Geometry check sheet. Reference: the model listing, model coordinates, mm. A direction names the side the tool comes from. Coordinates: 2 decimals unless noted, no trailing zeros. Order: outer loops, then holes, each group sorted by start corner. A loop starts at its lowest first (then second) coordinate and runs counter-clockwise, first axis right, second up. Notation, with made-up numbers: M -29.75,35 L -16.75,35 A22 ccw -16.75,56 Z; hole C 66,63.5 d11. An arc over 180 degrees is marked long. One line per item, written item: value. Start each with the question number.
1) Sectioned sample at D-D, the plane y = -1.5. Enter the section's corners in (x, z), then the cut area to 3 significant figures.
2) Draft check along Y on faces 1 (the flat face through (19, -22, 9.525)), 2 (the flat face through (32.6, -17.1, 11)), 3 (the flat face through (23.55, -3.13, 19.32)). Enter one of: pulls with the +Y half, pulls with the -Y half, needs draft (parallel to the pull), parting line crosses it, or undercut.
3) Sectioned sample at B-B, the plane x = 20.5. State how many separate pieces and enclosed holes the cut face has, then the cut area to 3 significant figures.
4) Thickness scan on L1, parallel to Y at x = 13, z = 27; L2, parallel to Y at x = 5, z = 23.5; L3, parallel to X at y = -16.5, z = 21. Record the ranges inside material, lowest first. Write a range as from..to.
5) Sectioned sample at C-C, the plane z = 35. Enter the section's corners in (x, y), then the cut area to 3 significant figures.
6) Sectioned sample at A-A, the plane z = 7.5. Enter the section's corners in (x, y), then the cut area to 3 significant figures.
7) Access from +Z, -Z, +X, -X, +Y, -Y to the whole of each face (thin tool, end or side, straight path). Record for faces 4 (the flat face through (28.423, -29.246, 25.856)), 5 (the flat face through (9.49, -32.45, 13.74)), 6 (the flat face through (17.285, -19.103, 22.874)), 7 (the flat face through (6, -21, 11)).
8) Go/stop test with flat-tipped pins: P1, Ø5.5, axis at x = 11, z = 20, coming from the -Y side; P2, Ø3.5, axis at y = -28.5, z = 27.5, coming from the -X side; P3, Ø1.5, axis at x = 29.5, y = -18.5, coming from the +Z side (3 decimals). Record where each tip stops, or that it passes through.
```python
from build123d import *

# Parameters (mm, degrees)
F0_W      = 38.1
F0_H      = 38.1
F1_DEPTH  = 38.1
F6_DEPTH  = 38.1
F8_DEPTH  = 38.1
F9_W      = 23.850204
F9_H      = 7.62
F9_W_2    = 24.289329
F10_DEPTH = 38.1


with BuildPart() as f1:
    # F0 (on Front) → F1 (new body)
    with BuildSketch(Plane.XZ):
        with Locations((19.05, 19.05)):
            Rectangle(F0_W, F0_H)
    extrude(amount=F1_DEPTH)

    # F5 (on offset) → F6 (cut)
    with BuildSketch(Plane.YZ.offset(38.1)):
        Polygon((-11.43, 13.264209), (-6.35, 38.1), (-9.257666, 38.1), (-31.75, 38.1), (-26.67, 13.264209), (-21.59, 28.575), (-16.51, 28.575), align=None)
        Polygon((-38.1, 0), (-31.75, 0), (-38.1, 38.1), align=None)
        Polygon((-25.4, 0), (-12.7, 0), (-19.05, 15.875), align=None)
        Polygon((-6.35, 0), (0, 0), (0, 38.1), align=None)
    extrude(amount=-F6_DEPTH, mode=Mode.SUBTRACT)

    # F7 (on offset) → F8 (cut)
    with BuildSketch(Plane.XZ.offset(38.1)):
        Polygon((0, 38.1), (0, 0), (6.35, 38.1), align=None)
        Polygon((19.05, 17.011538), (25.4, 38.1), (12.7, 38.1), align=None)
        Polygon((6.35, 0), (31.75, 0), (26.67, 22.225), (21.59, 9.525), (16.51, 9.525), (11.43, 22.225), align=None)
        Polygon((38.1, 0), (38.1, 38.1), (31.75, 38.1), align=None)
    extrude(amount=-F8_DEPTH, mode=Mode.SUBTRACT)

    # F9 (on offset) → F10 (cut)
    with BuildSketch(Plane.XY.offset(38.1)):
        with Locations((26.174898, -11.43)):
            Rectangle(F9_W, F9_H)
        with Locations((12.144664, -26.67)):
            Rectangle(F9_W_2, F9_H)
    extrude(amount=-F10_DEPTH, mode=Mode.SUBTRACT)


solid = f1.part
```
Final values:
1. outline: M 4.85,29.1 L 15.41,29.1 L 12.7,38.1 L 6.35,38.1 Z; M 22.69,29.1 L 33.25,29.1 L 31.75,38.1 L 25.4,38.1 Z
1. area: 152 mm^2
2. face 1: needs draft
2. face 2: undercut
2. face 3: pulls with the +Y half
3. separate pieces: 3
3. enclosed holes: 0
3. area: 173 mm^2
4. L1: y = -36.25..-30.48, -22.11..-15.99, -8.62..-1.85
4. L2: y = -35.67..-30.48, -22.86..-14.83, -9.34..-2.43
4. L3: x = 3.5..11.15, 11.92..17.85, 20.25..26.18, 26.95..34.6
5. outline: M 5.83,-37.58 L 13.63,-37.58 L 13.63,-31.12 L 5.83,-31.12 Z; M 5.83,-6.98 L 13.63,-6.98 L 13.63,-0.52 L 5.83,-0.52 Z; M 24.47,-37.58 L 32.27,-37.58 L 32.27,-31.12 L 24.47,-31.12 Z; M 24.47,-6.98 L 32.27,-6.98 L 32.27,-0.52 L 24.47,-0.52 Z
5. area: 202 mm^2
6. outline: M 1.25,-33 L 8.06,-33 L 8.06,-30.48 L 1.25,-30.48 Z; M 1.25,-22.86 L 8.06,-22.86 L 8.06,-22.4 L 1.25,-22.4 Z; M 1.25,-15.7 L 8.06,-15.7 L 8.06,-5.1 L 1.25,-5.1 Z; M 30.04,-33 L 36.85,-33 L 36.85,-22.4 L 30.04,-22.4 Z; M 30.04,-15.7 L 36.85,-15.7 L 36.85,-15.24 L 30.04,-15.24 Z; M 30.04,-7.62 L 36.85,-7.62 L 36.85,-5.1 L 30.04,-5.1 Z
6. area: 185 mm^2
7. face 4: +Z, +X, -X
7. face 5: -Z, +Y, -Y
7. face 6: +Z, +Y, -Y
7. face 7: -Z, +X, -X
8. P1: stops at y = -35.54
8. P2: stops at x = 24.29
8. P3: stops at z = 28.575
